Study the drawing (mm; zero at the part's minimum x, y, z) and answer. Give positions to 0.01 mm unless a question says otherwise; leave off trailing zeros. Order: outer loops, then holes, each group sorted by start corner. A loop starts at its lowest first (then second) coordinate and runs counter-clockwise, first axis right, second up.
Item 1: Find the intervals of material crossed by line 1 along Y through (x, z) = (26.5, 2.4); line 2 along X through (y, z) = (40, 1.5); line 3 along Y through (x, z) = (20, 3.9), in increasing order.
Item 2: Given pin 1 Ø8 at (x, y) = (33.5, 8.5) entering from +Z; pin 2 Ø2 at (y, z) = (47.5, 1.5) entering from +X; pin 3 Ø8 at (x, y) = (32, 47.5) entering from +Z; pin 4 Ø1.5 at (x, z) = (26, 1.5) entering from -Y, each flat-ended and moving along its own axis, determine where each tip first touches the part or whether it passes through.
Item 3: A cutting plane is placed at C-C (z = 0.75). Write down the section's boundary in (x, y), plus the area to 3 significant figures.
Item 4: The mould has two halves that part along Y. Classify the marked faces 1, 2 and 3: +Y half, -Y half, draft (parallel to the pull), parting line (faces both ways), or undercut.
Item 5: A cutting plane is placed at A-A (x = 26.5). Write down the section's boundary in (y, z), plus the area to 3 significant figures.
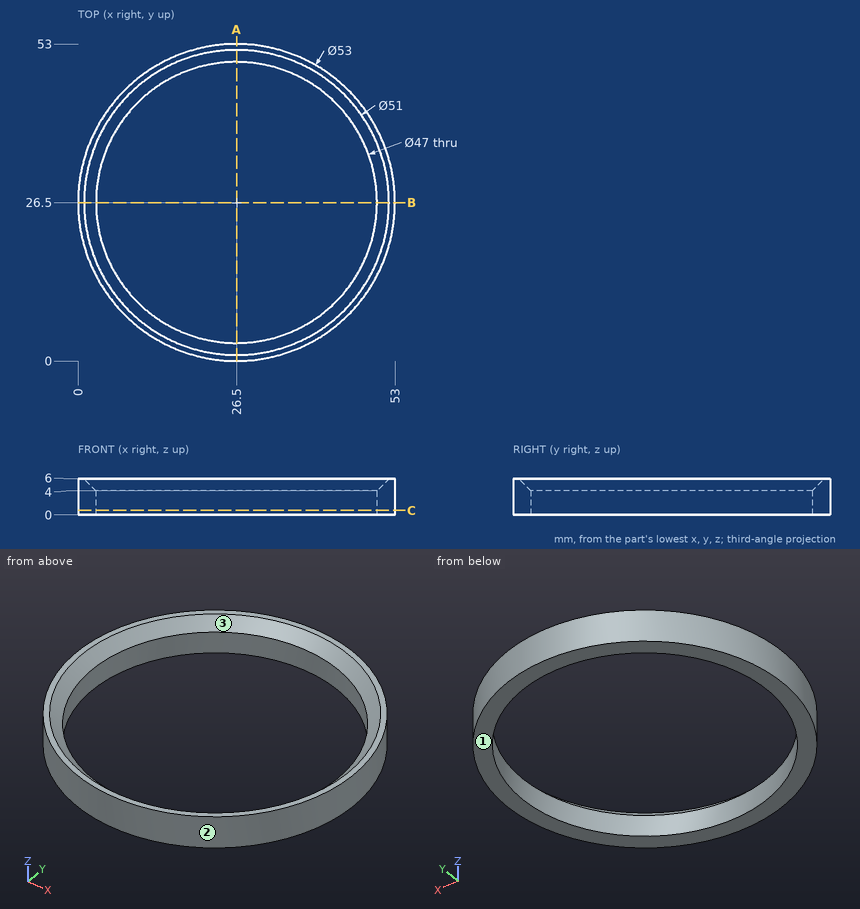
Response values:
1. line 1: y = 0 to 3, 50 to 53
1. line 2: x = 3.7 to 7.26, 45.74 to 49.3
1. line 3: y = 0.81 to 3.92, 49.08 to 52.19
2. pin 1: passes through
2. pin 2: stops at x = 43.89
2. pin 3: stops at z = 6
2. pin 4: stops at y = 0
3. outline: circle Ø53 at (26.5, 26.5); hole circle Ø47 at (26.5, 26.5)
3. area: 471 mm2
4. face 1: draft
4. face 2: parting line
4. face 3: undercut
5. outline: (0, 0) - (3, 0) - (3, 4) - (1, 6) - (0, 6) - close; (50, 0) - (53, 0) - (53, 6) - (52, 6) - (50, 4) - close
5. area: 32.0 mm2
